The listing builds one solid part. Answer for the finished solid, in the listing's coordinates (mm). Give positions to 0.01 mm unless a question says otherwise; leave off trailing zeros. Loops run counter-clockwise (first coordinate to the right, second up) from the corner with the lowest first, then second, coordinate; pieces in that order, holes last. Notation, with made-up numbers: (20, 75) - (71, 75) arc R7 ccw to (71, 86) - close; hole circle Ø10 at (31.25, 20). An arc over 180 degrees is marked (long way). Write item = value, one per line. Start each with the question number.
1) The mould has two halves that part along X. Classify faces 1 (the cylindrical face through (-0.1, -2.8, 0)), 2 (the cylindrical face through (-0.777, 2.832, -0.003)), 3 (the flat face through (-1, 2, 0.2)): +X half, -X half, draft (parallel to the pull), parting line (faces both ways), or undercut.
2) A flat-ended cylindrical pin translates along its axis: P1, Ø1.5, axis at x = -1.5, y = 0, coming from the -Z side. Find the tip coordinate at first contact, or state that the pin passes through.
3) The part is cut by section A-A on x = -1.2. Write down the section's boundary in (y, z).
4) Consider probe 1 along Y at (x, z) = (1.5, 0.05); probe 2 along Y at (x, z) = (0.9, -0.1); probe 3 along X at (y, z) = (-1.25, 0.1). Determine where each line is inside the solid, lowest interval first.
5) The part is cut by section C-C on y = -0.25. Write down the section's boundary in (x, z), plus the area to 3 significant figures.
6) The part is cut by section B-B on z = 0.1. Write down the section's boundary in (x, y), plus the area to 3 significant figures.
7) The part is cut by section D-D on y = 3. Write down the section's boundary in (x, z).
from build123d import *

# Parameters (mm, degrees)
SKETCH1_R           = 0.5
BOSS_EXTRUDE1_DEPTH = 0.2


with BuildPart() as part:
    # Sketch1 → Boss-Extrude1 (new, symmetric)
    with BuildSketch(Plane.XY):
        with BuildLine():
            Line((0.355177163, 4.066507215), (0.355177163, 1.866507215))
            ThreePointArc((0.355177163, 1.866507215), (0, -1.9), (-0.355177163, 1.866507215))
            Line((-0.355177163, 1.866507215), (-0.355177163, 4.066507215))
            ThreePointArc((-0.355177163, 4.066507215), (-1.128937663, 3.770726054), (-1.80338405, 3.289775039))
            ThreePointArc((-1.80338405, 3.289775039), (-2.114987451, 2.821889427), (-2.179084676, 2.263404717))
            ThreePointArc((-2.179084676, 2.263404717), (-2.179717367, 1.455750813), (-2.377239579, 0.67262234))
            ThreePointArc((-2.377239579, 0.67262234), (0, -2.8), (2.377239579, 0.67262234))
            ThreePointArc((2.377239579, 0.67262234), (2.179717367, 1.455750813), (2.179084676, 2.263404717))
            ThreePointArc((2.179084676, 2.263404717), (2.114987451, 2.821889427), (1.80338405, 3.289775039))
            ThreePointArc((1.80338405, 3.289775039), (1.128937663, 3.770726054), (0.355177163, 4.066507215))
        make_face()
        with Locations((-1.253673205, 2.682219999)):
            Circle(SKETCH1_R, mode=Mode.SUBTRACT)
        with Locations(Location((1.253673205, 2.682219999, 0), (0, 0, 180))):
            Circle(SKETCH1_R, mode=Mode.SUBTRACT)
    extrude(amount=BOSS_EXTRUDE1_DEPTH, both=True)


solid = part.part
Answer below:
q1.face_1 = parting line
q1.face_2 = undercut
q1.face_3 = draft
q2.P1 = -0.2
q3.outline = (-2.5, -0.2) - (-1.47, -0.2) - (-1.47, 0.2) - (-2.5, 0.2) - close; (1.47, -0.2) - (2.19, -0.2) - (2.19, 0.2) - (1.47, 0.2) - close; (3.18, -0.2) - (3.73, -0.2) - (3.73, 0.2) - (3.18, 0.2) - close
q4.probe_1 = -2.31 to -1.17, 1.17 to 2.25, 3.12 to 3.54
q4.probe_2 = -2.64 to -1.67, 1.67 to 2.33, 3.04 to 3.88
q4.probe_3 = -2.35 to -1.43, 1.43 to 2.35
q5.outline = (-2.55, -0.2) - (-1.88, -0.2) - (-1.88, 0.2) - (-2.55, 0.2) - close; (1.88, -0.2) - (2.55, -0.2) - (2.55, 0.2) - (1.88, 0.2) - close
q5.area = 0.533 mm2
q6.outline = (-2.38, 0.67) arc R2.55 ccw (long way) to (2.38, 0.67) arc R3.29 cw to (2.18, 2.26) arc R1.2 ccw to (1.8, 3.29) arc R3.27 ccw to (0.36, 4.07) - (0.36, 1.87) arc R1.9 cw (long way) to (-0.36, 1.87) - (-0.36, 4.07) arc R3.27 ccw to (-1.8, 3.29) arc R1.2 ccw to (-2.18, 2.26) arc R3.29 cw to start; hole circle Ø1 at (-1.25, 2.68); hole circle Ø1 at (1.25, 2.68)
q6.area = 13.6 mm2
q7.outline = (-2.03, -0.2) - (-1.64, -0.2) - (-1.64, 0.2) - (-2.03, 0.2) - close; (-0.87, -0.2) - (-0.36, -0.2) - (-0.36, 0.2) - (-0.87, 0.2) - close; (0.36, -0.2) - (0.87, -0.2) - (0.87, 0.2) - (0.36, 0.2) - close; (1.64, -0.2) - (2.03, -0.2) - (2.03, 0.2) - (1.64, 0.2) - close
